```python
from build123d import *

# Parameters (mm, degrees)
F0_R     = 88
F1_DEPTH = 30
F2_R     = 84
F3_DEPTH = 23
F4_R     = 1.5


# Not quite as in the source:
# - a feature names something its author has since deleted; it is built from what else it names


with BuildPart() as f1:
    # F0 (on Front) → F1 (new body)
    with BuildSketch(Plane.XZ):
        Circle(F0_R)
    extrude(amount=F1_DEPTH)

    # F2 (on face) → F3 (cut)
    with BuildSketch(Plane(origin=(0, 0, 0), x_dir=(-1, 0, 0), z_dir=(0, 1, 0))):
        Circle(F2_R)
    extrude(amount=-F3_DEPTH, mode=Mode.SUBTRACT)

    # F4
    f4_edges = [f1.edges().sort_by_distance(p)[0] for p in [
        (-88, -30, 0),
    ]]
    fillet(f4_edges, radius=F4_R)


solid = f1.part
```
Can you work these out from the model? Positions are in its coordinate system, mm. Coordinates: 2 decimals unless noted, no trailing zeros. Loops run counter-clockwise (first coordinate to the right, second up) from the corner with the lowest first, then second, coordinate; pieces in that order, holes last.
Item 1: Please list where these lines run through material, in increasing order: L1, parallel to Y at x = 46, z = -34; L2, parallel to X at y = -10.5, z = -78; L3, parallel to Z at x = -34.5, y = -8.
Answers below:
L1: y = -30 to -23
L2: x = -40.74 to -31.18, 31.18 to 40.74
L3: z = -80.96 to -76.59, 76.59 to 80.96
Item 2: Suppose I cut it at C-C (y = -13.5). Please give me the cut outline in (x, z), then the cut area to 3 significant figures.
Answers below:
outline: circle Ø176 at (0, 0); hole circle Ø168 at (0, 0)
area: 2,160 mm2
Item 3: Suppose I cut it at A-A (x = 0). Please give me the cut outline in (y, z).
Answers below:
outline: (-30, -86.5) arc R1.5 ccw to (-28.5, -88) - (0, -88) - (0, -84) - (-23, -84) - (-23, 84) - (0, 84) - (0, 88) - (-28.5, 88) arc R1.5 ccw to (-30, 86.5) - close
Item 4: Suppose I cut it at B-B (z = 0). Please give me the cut outline in (x, y), then the cut area to 3 significant figures.
Answers below:
outline: (-88, -28.5) arc R1.5 ccw to (-86.5, -30) - (86.5, -30) arc R1.5 ccw to (88, -28.5) - (88, 0) - (84, 0) - (84, -23) - (-84, -23) - (-84, 0) - (-88, 0) - close
area: 1,420 mm2
Item 5: If we mould it in two halves opening along Z, with no side actions, what happens to faces 1 (the face through (-19.077, -14.05, -85.907)), 2 (the face through (-80.12, -11.34, 25.23)), 3 (the face through (32, 0, -78)), 4 (the face through (1, -23, 1))? For each: released by +Z, released by -Z, zero draft, split by the parting line, or undercut.
Answers below:
face 1: split by the parting line
face 2: undercut
face 3: zero draft
face 4: undercut
Item 6: I'm going to push flat-ended pins straight in: pin 1 (3 mm diameter, centred on x = 13.5, y = -6.5, fed in from -Z); pin 2 (2 mm diameter, centred on x = 63.5, y = -11.5, fed in from -Z); pin 3 (10 mm diameter, centred on y = -7.5, z = -64.5, fed in from +X). Where does each tip first touch, or does it pass through?
Answers below:
pin 1: stops at z = -87.18
pin 2: stops at z = -61.95
pin 3: stops at x = 64.84
